Verification items for the finished model (mm, model axes). Round coordinates to 2 decimals unless told otherwise and drop trailing zeros. Write each loop counter-clockwise with the first axis right and the second up, starting at its lowest first coordinate (ties: lowest second). Pieces come first, ordered by that corner, then holes. Notation, with made-up numbers: M 64.5,60 L 106.5,60 A12 cw 106.5,74 Z; hole C 23.25,66 d1. An arc over 180 degrees is marked long. Answer in a Markdown table with one row per item. Add a question column.
1. Go/stop test with flat-tipped pins: pin 1 Ø1 at (x, z) = (-8.5, -34) entering from +Y; pin 2 Ø2 at (y, z) = (2, -118.5) entering from +X; pin 3 Ø0.7 at (x, z) = (-13, -151) entering from -Y. Record where each tip stops, or that it passes through.
2. Sectioned sample at B-B on z = -177. Record the cut outline in (x, y), plus the area to 3 significant figures.
3. Material ranges on probe 1 along X at (y, z) = (5.25, -171.5); probe 2 along Y at (x, z) = (-2, -166); probe 3 along X at (y, z) = (2.25, -60), recorded low to high.
4. Sectioned sample at A-A on y = 14.75. Record the cut outline in (x, z) (1 decimal).
```python
from build123d import *

# Parameters (mm, degrees)
EXTRUDE_THIN1_DEPTH = 206.375
FILLET1_R           = 1.016


with BuildPart() as part:
    # Sketch2 → Extrude-Thin1 (new body)
    with BuildSketch(Plane.XY):
        with BuildLine():
            Line((-10.715625, 0.396875), (-14.906625, 0))
            Line((-14.906625, 0), (-14.906625, 4.7625))
            Line((-14.906625, 4.7625), (-12.525255186, 4.7625))
            ThreePointArc((-12.525255186, 4.7625), (-11.617011589, 7.996272283), (-9.186204268, 10.314324348))
            ThreePointArc((-9.186204268, 10.314324348), (-5.372401066, 13.962420562), (-3.96875, 19.05))
            Line((-3.96875, 19.05), (-3.96875, 20.6375))
            Line((-3.96875, 20.6375), (0, 20.6375))
            Line((0, 20.6375), (-0.396875, 4.7625))
            Line((-0.396875, 4.7625), (-1.412557649, 4.787892066))
            Line((-1.412557649, 4.787892066), (-1.04171745, 19.6215))
            Line((-1.04171745, 19.6215), (-2.95275, 19.6215))
            Line((-2.95275, 19.6215), (-2.95275, 19.05))
            ThreePointArc((-2.95275, 19.05), (-4.500134936, 13.441452428), (-8.704471585, 9.419791161))
            ThreePointArc((-8.704471585, 9.419791161), (-10.986912369, 7.025809056), (-11.419137272, 3.7465))
            Line((-11.419137272, 3.7465), (-13.890625, 3.7465))
            Line((-13.890625, 3.7465), (-13.890625, 1.116757452))
            Line((-13.890625, 1.116757452), (-10.811408609, 1.408349913))
            Line((-10.811408609, 1.408349913), (-10.715625, 0.396875))
        make_face()
    extrude(amount=-EXTRUDE_THIN1_DEPTH)

    # Fillet1
    fillet1_edges = [part.edges().sort_by_distance(p)[0] for p in [
        (-11.419137272, 3.7465, -103.1875),
        (-14.906625, 0, -103.1875),
        (-14.906625, 4.7625, -103.1875),
        (-3.96875, 20.6375, -103.1875),
        (0, 20.6375, -103.1875),
    ]]
    fillet(fillet1_edges, radius=FILLET1_R)


solid = part.part
```
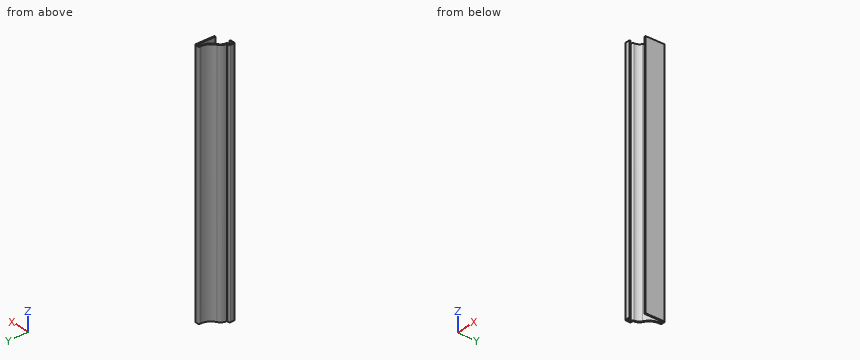
Geometry check:
| question | item | result |
|---|---|---|
| 1 | pin 1 | stops at y = 11.07 |
| 1 | pin 2 | stops at x = -10.77 |
| 1 | pin 3 | stops at y = 0.15 |
| 2 | outline | M -14.91,1.12 A1.02 ccw -13.79,0.11 L -10.72,0.4 L -10.81,1.41 L -13.89,1.12 L -13.89,3.75 L -12.53,3.75 A1.02 ccw -11.51,4.76 A5.33 cw -8.7,9.42 A10.94 ccw -2.95,19.05 L -2.95,19.62 L -1.04,19.62 L -1.41,4.79 L -0.4,4.76 L -0.03,19.6 A1.02 ccw -1.04,20.64 L -2.95,20.64 A1.02 ccw -3.97,19.62 L -3.97,19.05 A9.92 cw -9.19,10.31 A6.35 ccw -12.53,4.76 L -13.89,4.76 A1.02 ccw -14.91,3.75 Z |
| 2 | area | 46.7 mm2 |
| 3 | probe 1 | x = -12.5 to -11.48, -1.4 to -0.38 |
| 3 | probe 2 | y = 19.62 to 20.64 |
| 3 | probe 3 | x = -14.91 to -13.89 |
| 4 | outline | M -4.9,-206.4 L -3.8,-206.4 L -3.8,0 L -4.9,0 Z; M -1.2,-206.4 L -0.1,-206.4 L -0.1,0 L -1.2,0 Z |
